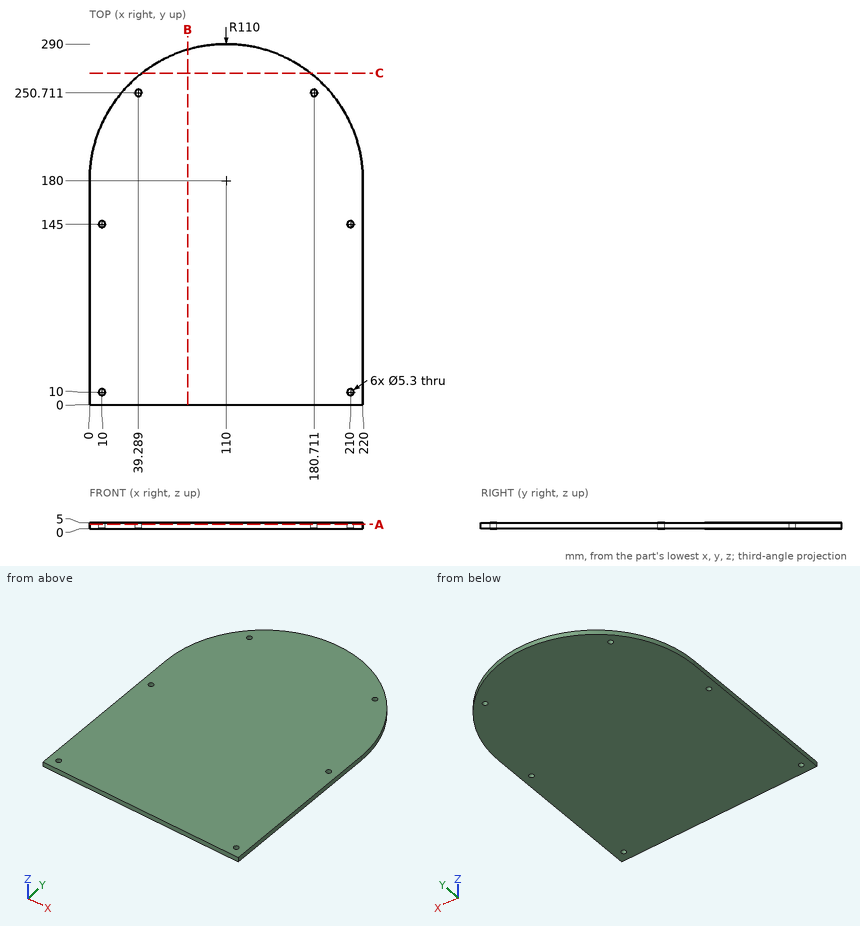
Geometry check sheet. Reference: drawing and pictorial views, mm from the part's lowest x, y, z. Round coordinates to 2 decimals unless told otherwise and drop trailing zeros. Loops run counter-clockwise (first coordinate to the right, second up) from the corner with the lowest first, then second, coordinate; pieces in that order, holes last. Notation, with made-up numbers: (86.25, 33.5) - (131.25, 33.5) arc R16 ccw to (131.25, 61.5) - close; hole circle Ø6 at (38.25, -19.75). An arc over 180 degrees is marked (long way). Use a Markdown table: item, result.
Q1. Go/stop test with flat-tipped pins: P1, Ø1, axis at y = 222.5, z = 0.5, coming from the +X side; P2, Ø3, axis at x = 39.5, z = 4.5, coming from the +Y side; P3, Ø1, axis at x = 23, z = 3, coming from the +Y side (1 decimal). Record where each tip stops, or that it passes through.
Solutions:
| item | result |
|---|---|
| P1 | stops at x = 211.67 |
| P2 | stops at y = 265.67 |
| P3 | stops at y = 248 |
Q2. Material ranges on line 1 (X direction, y = 145, z = 1.35); line 2 (X direction, y = 200.5, z = 4.45); line 3 (Y direction, x = 62, z = 0.4) (1 decimal), recorded low to high.
Solutions:
| item | result |
|---|---|
| line 1 | x = 0 to 7.35, 12.65 to 207.35, 212.65 to 220 |
| line 2 | x = 1.93 to 218.07 |
| line 3 | y = 0 to 279 |
Q3. Cross-section at A-A on z = 3.4. Record the cut outline in (x, y).
Solutions:
| item | result |
|---|---|
| outline | (0, 0) - (220, 0) - (220, 180) arc R110 ccw to (0, 180) - close; hole circle Ø5.3 at (10, 10); hole circle Ø5.3 at (10, 145); hole circle Ø5.3 at (39.29, 250.71); hole circle Ø5.3 at (180.71, 250.71); hole circle Ø5.3 at (210, 10); hole circle Ø5.3 at (210, 145) |
Q4. Cross-section at C-C on y = 266.5. Record the cut outline in (x, z).
Solutions:
| item | result |
|---|---|
| outline | (42.05, 0) - (177.95, 0) - (177.95, 5) - (42.05, 5) - close |
Q5. Cross-section at B-B on x = 79. Record the cut outline in (y, z).
Solutions:
| item | result |
|---|---|
| outline | (0, 0) - (285.54, 0) - (285.54, 5) - (0, 5) - close |
